```python
from build123d import *

# Parameters (mm, degrees)
BOSS_EXTRU_1_DEPTH      = 5
ESQUISSE2_W             = 8
ESQUISSE2_H             = 5
ESQUISSE2_W_2           = 15
ESQUISSE2_W_3           = 4.92
ESQUISSE2_H_2           = 65
ESQUISSE2_H_3           = 3
ESQUISSE2_H_4           = 15
ESQUISSE2_W_4           = 10
ESQUISSE2_W_5           = 25
ENL_V_MAT_EXTRU_1_DEPTH = 5
ESQUISSE3_W             = 7.280585373
ESQUISSE3_H             = 3.947256303
BOSS_EXTRU_2_DEPTH      = 5


with BuildPart() as part:
    # Esquisse1 → Boss.-Extru.1 (new body)
    with BuildSketch(Plane.XY):
        with BuildLine():
            Line((0, 0), (80, 0))
            Line((80, 0), (80, 17.15))
            Line((80, 17.15), (49.330858803, 17.15))
            Line((49.330858803, 17.15), (49.330858803, 25.109342079))
            add(Edge.make_bspline(
                [(80, 59.779072791), (49.330858803, 55.600211761), (49.330858803, 25.109342079)],
                knots=[1.708281914, 1.708281914, 1.708281914, 3.141592654, 3.141592654, 3.141592654], degree=2, weights=[1, 0.754006918, 1]))
            Line((80, 59.779072791), (80, 270))
            Line((80, 270), (0, 270))
            Line((0, 270), (0, 0))
        make_face()
    extrude(amount=BOSS_EXTRU_1_DEPTH)

    # Esquisse2 → Enlèv. mat.-Extru.1 (cut)
    with BuildSketch(Plane.XY.offset(5)):
        with Locations((55.679721659, 99.250434868)):
            Rectangle(ESQUISSE2_W, ESQUISSE2_H)
        Polygon((75.08, 12.15), (70, 12.15), (70, 17.15), (80, 17.15), (80, 3), (75.08, 3), align=None)
        with Locations((45, 14.65)):
            Rectangle(ESQUISSE2_W_2, ESQUISSE2_H)
        with Locations((7.5, 14.65)):
            Rectangle(ESQUISSE2_W_2, ESQUISSE2_H)
        with Locations((77.54, 98.5)):
            Rectangle(ESQUISSE2_W_3, ESQUISSE2_H_2)
        with Locations((2.46, 1.5)):
            Rectangle(ESQUISSE2_W_3, ESQUISSE2_H_3)
        with Locations((77.54, 183.5)):
            Rectangle(ESQUISSE2_W_3, ESQUISSE2_H_4)
        with Locations((77.54, 153.5)):
            Rectangle(ESQUISSE2_W_3, ESQUISSE2_H_4)
        with Locations((77.54, 213.5)):
            Rectangle(ESQUISSE2_W_3, ESQUISSE2_H_4)
        with Locations((77.54, 243.5)):
            Rectangle(ESQUISSE2_W_3, ESQUISSE2_H_4)
        with Locations((77.54, 273.5)):
            Rectangle(ESQUISSE2_W_3, ESQUISSE2_H_4)
        with Locations((2.46, 273.5)):
            Rectangle(ESQUISSE2_W_3, ESQUISSE2_H_4)
        with Locations((2.46, 243.5)):
            Rectangle(ESQUISSE2_W_3, ESQUISSE2_H_4)
        with Locations((2.46, 213.5)):
            Rectangle(ESQUISSE2_W_3, ESQUISSE2_H_4)
        with Locations((2.46, 183.5)):
            Rectangle(ESQUISSE2_W_3, ESQUISSE2_H_4)
        with Locations((2.46, 153.5)):
            Rectangle(ESQUISSE2_W_3, ESQUISSE2_H_4)
        with Locations((2.46, 123.5)):
            Rectangle(ESQUISSE2_W_3, ESQUISSE2_H_4)
        with Locations((2.46, 93.5)):
            Rectangle(ESQUISSE2_W_3, ESQUISSE2_H_4)
        with Locations((2.46, 63.5)):
            Rectangle(ESQUISSE2_W_3, ESQUISSE2_H_4)
        with Locations((2.46, 33.5)):
            Rectangle(ESQUISSE2_W_3, ESQUISSE2_H_4)
        with Locations((15, 267.5)):
            Rectangle(ESQUISSE2_W_4, ESQUISSE2_H)
        with Locations((47.5, 267.5)):
            Rectangle(ESQUISSE2_W_5, ESQUISSE2_H)
    extrude(amount=-ENL_V_MAT_EXTRU_1_DEPTH, mode=Mode.SUBTRACT)

    # Esquisse3 → Boss.-Extru.2 (add)
    with BuildSketch(Plane(origin=(0, 0, 0), x_dir=(-1, 0, 0), z_dir=(0, 0, -1))):
        with Locations((-76.359707313, 59.973628152)):
            Rectangle(ESQUISSE3_W, ESQUISSE3_H)
    extrude(amount=-BOSS_EXTRU_2_DEPTH)


solid = part.part
```
CAD build for the part. Positions are in the model's coordinates, mm. A direction names the side the tool comes from. Coordinates: 2 decimals unless noted, no trailing zeros. Order: outer loops, then holes, each group sorted by start corner. A loop starts at its lowest first (then second) coordinate and runs counter-clockwise, first axis right, second up. Notation, with made-up numbers: M 79.5,18 L 89.5,18 A6 cw 89.5,26 Z; hole C -27.75,-24 d8. An arc over 180 degrees is marked long. Write each question's results on one line, items separated by ' | '. Start each with the question number.
Q1. Cut at A-A (x = 46). List the corners of the cut face in (y, z).
Q2. Which spindle directions (+Z, -Z, +X, -X, +Y, -Y) get a long thin tool onto all of the face, cutting with end or side? Do faces 4 (the flat face through (4.92, 243, 3)), 5 (the flat face through (75.08, 8, 3)), 6 (the flat face through (20, 267, 3)). Say none if no direction does.
Q3. Cut at B-B (y = 125.5). List the corners of the cut face in (x, z).
Q4. Flat gauge pins, fed straight in: P1, Ø1.5, axis at y = 77.5, z = 2.5, coming from the +X side; P2, Ø3, axis at x = 42, z = 4, coming from the +Y side; P3, Ø2.5, axis at y = 211, z = 2, coming from the -X side. Where does each tip first touch, or does it go through?
Q5. Drill centre lines: probe 1 along X at (y, z) = (97.5, 1.7); probe 2 along Y at (x, z) = (55, 3); probe 3 along Y at (x, z) = (10.5, 3.85). Where is each one in solid material? Low to high. Write a range as from..to.
Q6. Pull direction Y, two halves, no side cores. Call faces 1 (the flat face through (10, 267, 3)), 2 (the flat face through (59.68, 99, 3)), 3 (the flat face through (42, 0, 2)): +Y half, -Y half, draft (parallel to the pull), parting line (faces both ways), or undercut.
Found:
1) outline: M 0,0 L 12.15,0 L 12.15,5 L 0,5 Z; M 17.15,0 L 265,0 L 265,5 L 17.15,5 Z
2) face 4: +Z, -Z, -X | face 5: +Z, -Z, +X | face 6: +Z, -Z, +Y
3) outline: M 4.92,0 L 75.08,0 L 75.08,5 L 4.92,5 Z
4) P1: x = 75.08 | P2: y = 265 | P3: x = 4.92
5) probe 1: 4.92..51.68, 59.68..75.08 | probe 2: 0..17.15, 44.07..96.75, 101.75..265 | probe 3: 0..12.15, 17.15..265
6) face 1: draft | face 2: undercut | face 3: -Y half
